Work out the finished part from the listing and answer in its coordinate system (mm). Coordinates: 2 decimals unless noted, no trailing zeros. Loops run counter-clockwise (first coordinate to the right, second up) from the corner with the lowest first, then second, coordinate; pieces in that order, holes last. Notation, with made-up numbers: (81.5, 28.5) - (123.5, 28.5) arc R20 ccw to (123.5, 60.5) - close; hole circle Ø1 at (17, -35). An arc over 180 degrees is marked (long way). Write each question's results on one line, items separated by ' | '. Start each with the question number.
Item 1: Section C-C, the plane z = -2 is taken. Write down the section's boundary in (x, y).
Item 2: Section A-A, the plane x = 61 is taken. Write down the section's boundary in (y, z), plus the area to 3 significant figures.
Item 3: Section B-B, the plane y = 49 is taken. Write down the section's boundary in (x, z), plus the area to 3 significant figures.
Item 4: Consider probe 1 along X at (y, z) = (61.5, -35.1); probe 2 along X at (y, z) = (49, 92.5); probe 3 along Y at (x, z) = (1, -20.5). Determine where each line is inside the solid, lowest interval first. Write a range as [from, to].
Item 5: Each of these flat-tipped pins is pushed along its axis until it touches: pin 1 Ø3.5 at (x, y) = (9.4, 61.5) entering from -Z; pin 2 Ø3 at (x, y) = (9, 20.5) entering from +Z. Where does it stop, or does it pass through?
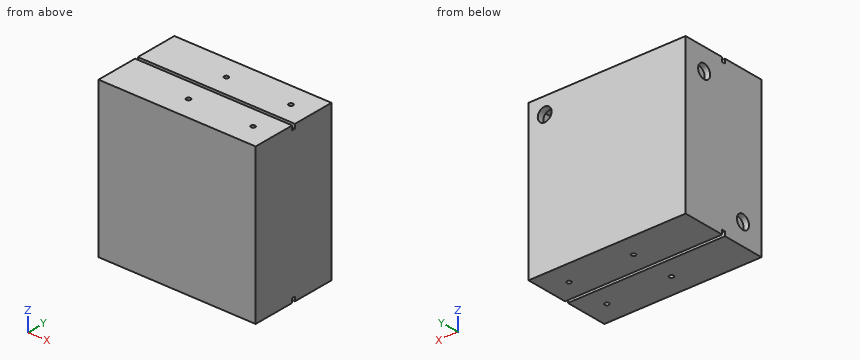
from build123d import *

# Parameters (mm, degrees)
SKETCH1_W           = 146
SKETCH1_H           = 144
BOSS_EXTRUDE1_DEPTH = 82
SHELL1_T            = 6
SKETCH2_R           = 6.45
CUT_EXTRUDE1_DEPTH  = 10
SKETCH3_R           = 6.5
CUT_EXTRUDE2_DEPTH  = 5
SKETCH4_W           = 4
SKETCH4_H           = 3
CUT_EXTRUDE3_DEPTH  = 199.806250042
SKETCH5_R           = 2
CUT_EXTRUDE4_DEPTH  = 4
CUT_EXTRUDE5_START  = -4
SKETCH6_R           = 2
CUT_EXTRUDE5_DEPTH  = 4


with BuildPart() as part:
    # Sketch1 → Boss-Extrude1 (new body)
    with BuildSketch(Plane(origin=(0, 0, 0), x_dir=(1, 0, 0), z_dir=(0, 1, 0))):
        with Locations((16.396923077, -35.163076923)):
            Rectangle(SKETCH1_W, SKETCH1_H)
    extrude(amount=BOSS_EXTRUDE1_DEPTH)

    # Shell1 (no face opened: a closed hollow body)
    add(offset(amount=-SHELL1_T, mode=Mode.PRIVATE), mode=Mode.SUBTRACT)

    # Sketch2 → Cut-Extrude1 (cut)
    with BuildSketch(Plane(origin=(0, 82, 0), x_dir=(1, 0, 0), z_dir=(0, 1, 0))):
        with Locations(Location((74.396923077, -92.163076923, 0), (0, 0, 270))):
            Circle(SKETCH2_R)
    extrude(amount=-CUT_EXTRUDE1_DEPTH, mode=Mode.SUBTRACT)

    # Sketch3 → Cut-Extrude2 (cut)
    with BuildSketch(Plane.ZY.offset(56.603076923)):
        with Locations((87.163076923, 62)):
            Circle(SKETCH3_R)
        with Locations((-16.836923077, 20)):
            Circle(SKETCH3_R)
    extrude(amount=-CUT_EXTRUDE2_DEPTH, mode=Mode.SUBTRACT)

    # Sketch4 → Cut-Extrude3 (cut, through all)
    with BuildSketch(Plane.ZY.offset(56.603076923)):
        with Locations((-34.836923077, 41)):
            Rectangle(SKETCH4_W, SKETCH4_H)
        with Locations((105.163076923, 41)):
            Rectangle(SKETCH4_W, SKETCH4_H)
    extrude(amount=-CUT_EXTRUDE3_DEPTH, mode=Mode.SUBTRACT)

    # Sketch5 → Cut-Extrude4 (cut)
    with BuildSketch(Plane.XY.offset(107.163076923)):
        with Locations((69.396923077, 61.5)):
            Circle(SKETCH5_R)
        with Locations((9.396923077, 61.5)):
            Circle(SKETCH5_R)
        with Locations((9.396923077, 20.5)):
            Circle(SKETCH5_R)
        with Locations((69.396923077, 20.5)):
            Circle(SKETCH5_R)
    extrude(amount=-CUT_EXTRUDE4_DEPTH, mode=Mode.SUBTRACT)

    # Sketch6 → Cut-Extrude5 (cut)
    with BuildSketch(Plane(origin=(0, 0, -36.836923077), x_dir=(-1, 0, 0), z_dir=(0, 0, -1)).offset(CUT_EXTRUDE5_START)):
        with Locations(Location((-9.396923077, 61.5, 0), (0, 0, 180))):
            Circle(SKETCH6_R)
        with Locations(Location((-69.396923077, 61.5, 0), (0, 0, 180))):
            Circle(SKETCH6_R)
        with Locations(Location((-69.396923077, 20.5, 0), (0, 0, 180))):
            Circle(SKETCH6_R)
        with Locations(Location((-9.396923077, 20.5, 0), (0, 0, 180))):
            Circle(SKETCH6_R)
    extrude(amount=CUT_EXTRUDE5_DEPTH, mode=Mode.SUBTRACT)


solid = part.part
Answer key:
1) outline: (-56.6, 0) - (89.4, 0) - (89.4, 82) - (-56.6, 82) - close; hole (-50.6, 6) - (83.4, 6) - (83.4, 76) - (-50.6, 76) - close
2) outline: (0, -36.84) - (39.5, -36.84) - (39.5, -32.84) - (42.5, -32.84) - (42.5, -36.84) - (82, -36.84) - (82, 107.16) - (42.5, 107.16) - (42.5, 103.16) - (39.5, 103.16) - (39.5, 107.16) - (0, 107.16) - close; hole (6, -30.84) - (76, -30.84) - (76, 101.16) - (6, 101.16) - close | area: 2,540 mm^2
3) outline: (-56.6, -36.84) - (89.4, -36.84) - (89.4, 107.16) - (-56.6, 107.16) - close; hole (-50.6, -30.84) - (83.4, -30.84) - (83.4, 101.16) - (-50.6, 101.16) - close | area: 3,340 mm^2
4) probe 1: x = [-56.6, 7.4], [11.4, 67.4], [71.4, 89.4] | probe 2: x = [-56.6, -50.6], [83.4, 89.4] | probe 3: y = [0, 6], [76, 82]
5) pin 1: stops at z = -32.84 | pin 2: stops at z = 103.16
